Geometry check sheet. Reference: the model listing, model coordinates, mm. Face numbers are marked on the shaded views. A direction names the side the tool comes from. Give positions to 0.01 mm unless a question says otherwise; leave off trailing zeros. Loops run counter-clockwise (first coordinate to the right, second up) from the corner with the lowest first, then second, coordinate; pieces in that order, holes last. Notation, with made-up numbers: (-3.5, 20) -> (32.5, 20) arc R14 cw to (32.5, 47) -> close; hole circle Ø2 at (61, 49). An arc over 180 degrees is marked (long way). Write each question's results on one line, items separated by ' | '. Start each with the question number.
1) Set-up check for the marked faces 1 and 2: record each of +Z, -Z, +X, -X, +Y, -Y from which the full face is reachable in a straight line by a thin tool's end or side.
2) Draft check along Z on the marked faces 3, 4 and 5. Enter one of: pulls with the +Z half, pulls with the -Z half, needs draft (parallel to the pull), parting line crosses it, or undercut.
3) Sectioned sample at C-C on x = 14. Record the cut outline in (y, z), then the cut area to 3 significant figures.
4) Sectioned sample at B-B on z = 0. Record the cut outline in (x, y), then the cut area to 3 significant figures.
5) Sectioned sample at A-A on y = 0. Record the cut outline in (x, z), then the cut area to 3 significant figures.
6) Depth check by flat-ended pin: pin 1 (18 mm diameter, centred on y = 0, z = 0, fed in from +X); pin 2 (4 mm diameter, centred on x = -12, z = -7.5, fed in from +Y); pin 3 (8 mm diameter, centred on x = 12, y = -12.5, fed in from -Z); pin 4 (2 mm diameter, centred on x = 0, y = -17.5, fed in from +Z). Enter the tip coordinate at first touch or a pass-through.
7) Scan lines: line 1 (Y direction, x = 0, z = 19); line 2 (X direction, y = -3, z = -16); line 3 (Y direction, x = -5.5, z = 2.5). Record each from-to range of solid material in increasing order. Write a range as from..to.
```python
from build123d import *

# Parameters (mm, degrees)
SKETCH1_R                       = 13
BOSS_EXTRUDE1_DEPTH             = 17
SKETCH2_R                       = 26.5
BOSS_EXTRUDE2_DEPTH             = 1
CHAMFER1_SIZE                   = 0.5
SKETCH4_R                       = 2.5
WYTNIJ_WYCI_GNI_CIE1_DEPTH      = 18
WYTNIJ_WYCI_GNI_CIE1_DEPTH_BACK = 2
SKETCH1_3_R                     = 13
DODANIE_WYCI_GNI_CIE1_DEPTH     = 18
SZKIC5_R                        = 10
WYTNIJ_WYCI_GNI_CIE2_DEPTH      = 40
WYTNIJ_WYCI_GNI_CIE3_DEPTH      = 40
SFAZOWANIE1_SIZE                = 0.5
ZAOKR_GLENIE1_R                 = 1
SZKIC7_W                        = 25
SZKIC7_H                        = 18.250813048
WYTNIJ_WYCI_GNI_CIE4_DEPTH      = 10
ZAOKR_GLENIE2_R                 = 1


with BuildPart() as part:
    # Sketch1 → Boss-Extrude1 (new body)
    with BuildSketch(Plane(origin=(0, 0, 0), x_dir=(0, 0, -1), z_dir=(1, 0, 0))):
        Circle(SKETCH1_R)
    extrude(amount=BOSS_EXTRUDE1_DEPTH)

    # Sketch2 → Boss-Extrude2 (add, symmetric)
    with BuildSketch(Plane(origin=(0, 0, 0), x_dir=(0, 0, -1), z_dir=(1, 0, 0))):
        Circle(SKETCH2_R)
    extrude(amount=BOSS_EXTRUDE2_DEPTH, both=True)

    # Chamfer1
    chamfer1_edges = [part.edges().sort_by_distance(p)[0] for p in [
        (17, 0, 13),
        (-1, 0, 26.5),
        (1, 0, 26.5),
    ]]
    chamfer(chamfer1_edges, length=CHAMFER1_SIZE)

    # Sketch4 → Wytnij-wyci_gni_cie1 (cut, two sides)
    with BuildSketch(Plane(origin=(0, 0, 0), x_dir=(0, 0, -1), z_dir=(1, 0, 0))) as wytnij_wyci_gni_cie1_sk:
        with Locations((17.219847954, -8.029746973)):
            Circle(SKETCH4_R)
        with Locations((-19, 0)):
            Circle(SKETCH4_R)
        with Locations((14.554844419, 12.212964584)):
            Circle(SKETCH4_R)
        with Locations((0, 19)):
            Circle(SKETCH4_R)
        with Locations((-17.854159795, -6.498382723)):
            Circle(SKETCH4_R)
        with Locations((-16.454482672, 9.5)):
            Circle(SKETCH4_R)
        with Locations((18.711347307, 3.299315376)):
            Circle(SKETCH4_R)
        with Locations((-12.212964584, 14.554844419)):
            Circle(SKETCH4_R)
        with Locations((9.5, 16.454482672)):
            Circle(SKETCH4_R)
    extrude(amount=WYTNIJ_WYCI_GNI_CIE1_DEPTH, mode=Mode.SUBTRACT)
    extrude(wytnij_wyci_gni_cie1_sk.sketch, amount=-WYTNIJ_WYCI_GNI_CIE1_DEPTH_BACK, mode=Mode.SUBTRACT)

    # Sketch1_3 → Dodanie-wyci_gni_cie1 (add)
    with BuildSketch(Plane(origin=(0, 0, 0), x_dir=(0, 0, -1), z_dir=(1, 0, 0))):
        Circle(SKETCH1_3_R)
    extrude(amount=-DODANIE_WYCI_GNI_CIE1_DEPTH)

    # Szkic5 → Wytnij-wyci_gni_cie2 (cut)
    with BuildSketch(Plane(origin=(17, 0, 0), x_dir=(0, 0, -1), z_dir=(1, 0, 0))):
        Circle(SZKIC5_R)
    extrude(amount=-WYTNIJ_WYCI_GNI_CIE2_DEPTH, mode=Mode.SUBTRACT)

    # Szkic4 → Wytnij-wyci_gni_cie3 (cut)
    with BuildSketch(Plane.ZY.offset(1)):
        with BuildLine():
            Line((18, -15.874507866), (18, -28.40570104))
            Line((18, -28.40570104), (34.562586152, -28.40570104))
            Line((34.562586152, -28.40570104), (34.562586152, 27.915934969))
            Line((34.562586152, 27.915934969), (-37.904902175, 28.979399158))
            Line((-37.904902175, 28.979399158), (-37.904902175, -27.460164602))
            Line((-37.904902175, -27.460164602), (-18, -25.464511286))
            Line((-18, -25.464511286), (-18, -15.874507866))
            ThreePointArc((-18, -15.874507866), (0, 24), (18, -15.874507866))
        make_face()
    extrude(amount=-WYTNIJ_WYCI_GNI_CIE3_DEPTH, mode=Mode.SUBTRACT)

    # Sfazowanie1
    sfazowanie1_edges = [part.edges().sort_by_distance(p)[0] for p in [
        (-18, 0, 13),
    ]]
    chamfer(sfazowanie1_edges, length=SFAZOWANIE1_SIZE)

    # Zaokr_glenie1
    zaokr_glenie1_edges = [part.edges().sort_by_distance(p)[0] for p in [
        (-1, 0, 13),
        (1, 0, 13),
    ]]
    fillet(zaokr_glenie1_edges, radius=ZAOKR_GLENIE1_R)

    # Szkic7 → Wytnij-wyci_gni_cie4 (cut)
    with BuildSketch(Plane.ZY.offset(1)):
        with Locations((0, -24.125406524)):
            Rectangle(SZKIC7_W, SZKIC7_H)
    extrude(amount=-WYTNIJ_WYCI_GNI_CIE4_DEPTH, mode=Mode.SUBTRACT)

    # Zaokr_glenie2
    zaokr_glenie2_edges = [part.edges().sort_by_distance(p)[0] for p in [
        (0, -15.874507866, 18),
        (0, -15.874507866, -18),
    ]]
    fillet(zaokr_glenie2_edges, radius=ZAOKR_GLENIE2_R)


solid = part.part
```
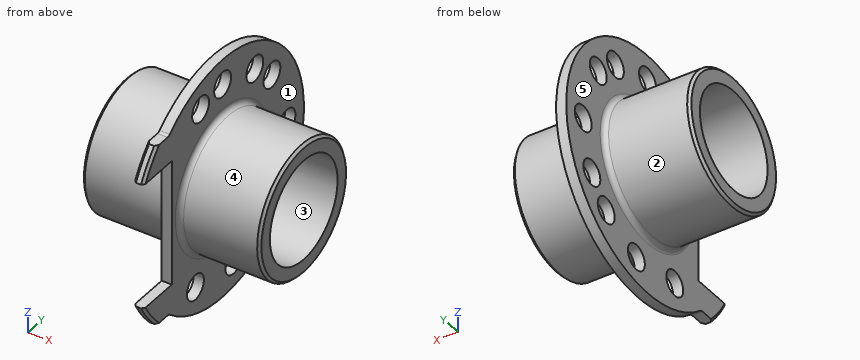
Result:
1) face 1: +X | face 2: -X
2) face 3: undercut | face 4: parting line crosses it | face 5: needs draft
3) outline: circle Ø26 at (0, 0); hole circle Ø20 at (0, 0) | area: 217 mm^2
4) outline: (-18, -12.5) -> (-17.5, -13) -> (-2, -13) arc R1 cw to (-1, -14) -> (-1, -15) -> (1, -15) -> (1, -14) arc R1 cw to (2, -13) -> (16.5, -13) -> (17, -12.5) -> (17, -10) -> (-18, -10) -> close; (-18, 10) -> (17, 10) -> (17, 12.5) -> (16.5, 13) -> (2, 13) arc R1 cw to (1, 14) -> (1, 16.5) -> (-1, 16.5) -> (-1, 14) arc R1 cw to (-2, 13) -> (-17.5, 13) -> (-18, 12.5) -> close; (-1, 21.5) -> (1, 21.5) -> (1, 24) -> (-1, 24) -> close | area: 226 mm^2
5) outline: (-18, -12.5) -> (-17.5, -13) -> (-2, -13) arc R1 cw to (-1, -14) -> (-1, -24) -> (1, -24) -> (1, -14) arc R1 cw to (2, -13) -> (16.5, -13) -> (17, -12.5) -> (17, -10) -> (-18, -10) -> close; (-18, 10) -> (17, 10) -> (17, 12.5) -> (16.5, 13) -> (2, 13) arc R1 cw to (1, 14) -> (1, 16.5) -> (-1, 16.5) -> (-1, 14) arc R1 cw to (-2, 13) -> (-17.5, 13) -> (-18, 12.5) -> close; (-1, 21.5) -> (1, 21.5) -> (1, 24) -> (-1, 24) -> close | area: 244 mm^2
6) pin 1: through | pin 2: y = 11.78 | pin 3: z = -9.84 | pin 4: z = 18
7) line 1: -14.66..-8.72, -4.28..-2.5, 2.5..14.66 | line 2: -1..1 | line 3: -12.76..-9.68, 9.68..12.76
